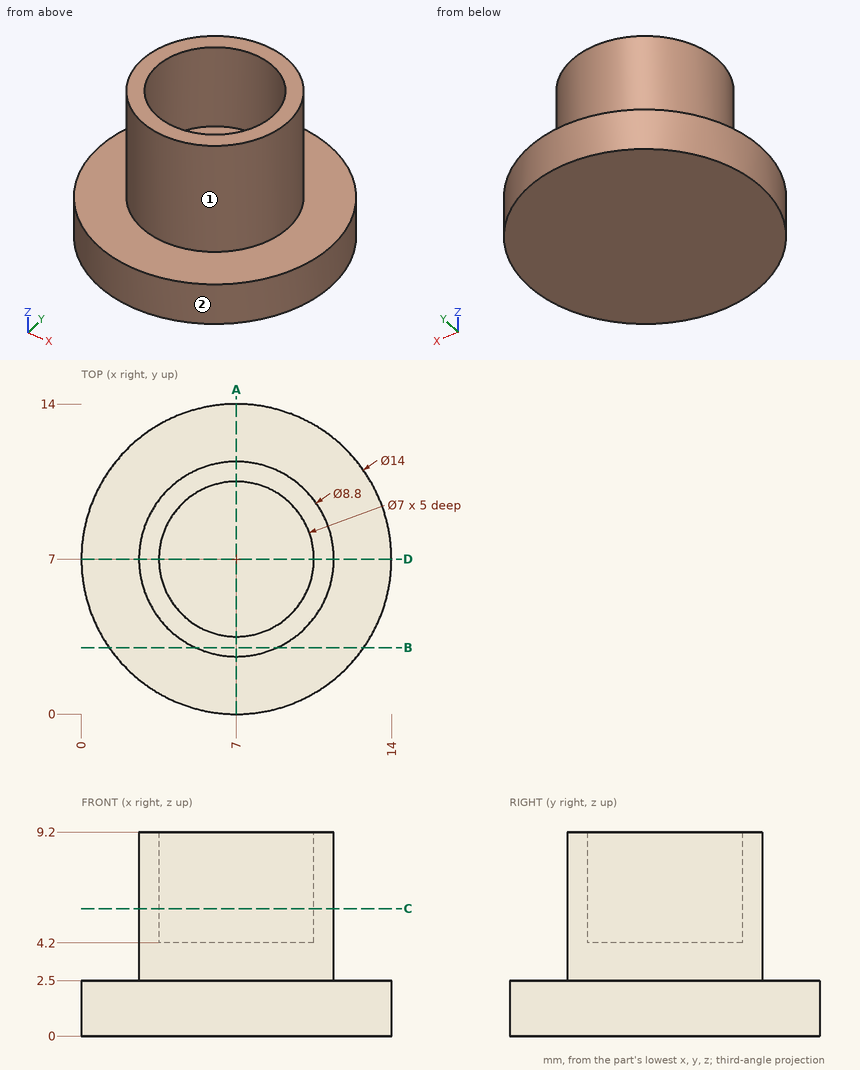
Check sheet for the drawn part. Datum: minimum x, y, z corner. Units: mm. A direction names the side the tool comes from. Round coordinates to 2 decimals unless told otherwise and drop trailing zeros. Order: outer loops, then holes, each group sorted by start corner. A loop starts at its lowest first (then second) coordinate and runs counter-clockwise, first axis right, second up.
(1) Scan lines: probe 1 along Y at (x, z) = (7, 5.4); probe 2 along Z at (x, y) = (3, 4.5); probe 3 along Z at (x, y) = (9.25, 6.25). Record each from-to range of solid material in increasing order.
(2) Go/stop test with flat-tipped pins: P1, Ø1, axis at y = 8.5, z = 4, coming from the -X side; P2, Ø6, axis at x = 2.5, y = 6, coming from the -Z side; P3, Ø3.5, axis at x = 7.5, y = 7, coming from the +Z side; P4, Ø1.5, axis at x = 11, z = 4, coming from the +Y side. Record where each tip stops, or that it passes through.
(3) Cross-section at A-A, the plane x = 7. Enter the section's corners in (y, z).
(4) Access from +Z, -Z, +X, -X, +Y, -Y to the whole of each face (thin tool, end or side, straight path). Record for the marked faces 1 and 2.
(5) Cross-section at B-B, the plane y = 3. Enter the section's corners in (x, z).
(6) Cross-section at C-C, the plane z = 5.75. Enter the section's corners in (x, y), and give its area (3 significant figures).
Check sheet entries:
1. probe 1: y = 2.6 to 3.5, 10.5 to 11.4
1. probe 2: z = 0 to 2.5
1. probe 3: z = 0 to 4.2
2. P1: stops at x = 2.72
2. P2: stops at z = 0
2. P3: stops at z = 4.2
2. P4: stops at y = 9.97
3. outline: (0, 0) - (14, 0) - (14, 2.5) - (11.4, 2.5) - (11.4, 9.2) - (10.5, 9.2) - (10.5, 4.2) - (3.5, 4.2) - (3.5, 9.2) - (2.6, 9.2) - (2.6, 2.5) - (0, 2.5) - close
4. face 1: +Z
4. face 2: +Z, -Z
5. outline: (1.26, 0) - (12.74, 0) - (12.74, 2.5) - (8.83, 2.5) - (8.83, 9.2) - (5.17, 9.2) - (5.17, 2.5) - (1.26, 2.5) - close
6. outline: circle Ø8.8 at (7, 7); hole circle Ø7 at (7, 7)
6. area: 22.3 mm2
